For this review, use the dimensioned drawing (mm, ordinates from the lowest corner) and the shaded views. A direction names the side the tool comes from. Coordinates: 2 decimals unless noted, no trailing zeros. Loops run counter-clockwise (first coordinate to the right, second up) from the corner with the lowest first, then second, coordinate; pieces in that order, holes last. Notation, with made-up numbers: (6.5, 55.25) - (20.5, 55.25) arc R28 ccw to (20.5, 94.25) - close; hole circle Ø6 at (-13.5, -22.75). An arc over 180 degrees is marked (long way). Answer in a Markdown table with one row per item. Add a question column.
(1) We need section D-D on x = 12.5. Write out the cut boundary in (y, z), plus the area to 3 significant figures.
(2) For line 1 along X through (y, z) = (10, 34); line 2 along Z through (x, y) = (22.75, 9.75); line 3 along Z through (x, y) = (17.25, 8), list the stretches that pass through material, from the lowest coordinate up.
(3) We need section A-A on z = 32. Write out the cut boundary in (x, y).
(4) We need section C-C on y = 12.5. Write out the cut boundary in (x, z), plus the area to 3 significant figures.
(5) Machinability: for the marked faces 1, 2, 3, 4 and 5, which of the approach directions +Z, -Z, +X, -X, +Y, -Y give a long, thin tool a straight path to every point of the face, cutting with its end or side? Answer none if there is none.
(6) Mouldability with a two-part tool opening along Z and no side actions: class the marked faces 6, 7, 8 and 9 as +Z half, -Z half, draft (parallel to the pull), parting line (faces both ways), or undercut.
(7) For P1, Ø2, axis at x = 20.5, z = 6, coming from the +Y side; P2, Ø2, axis at y = 11, z = 21, coming from the +X side; P3, Ø5.5, axis at y = 14, z = 34.5, coming from the +X side, all flat-tipped, find the tip position at first contact; note any pin that passes through.
(8) We need section B-B on x = 4. Write out the cut boundary in (y, z), plus the area to 3 significant figures.
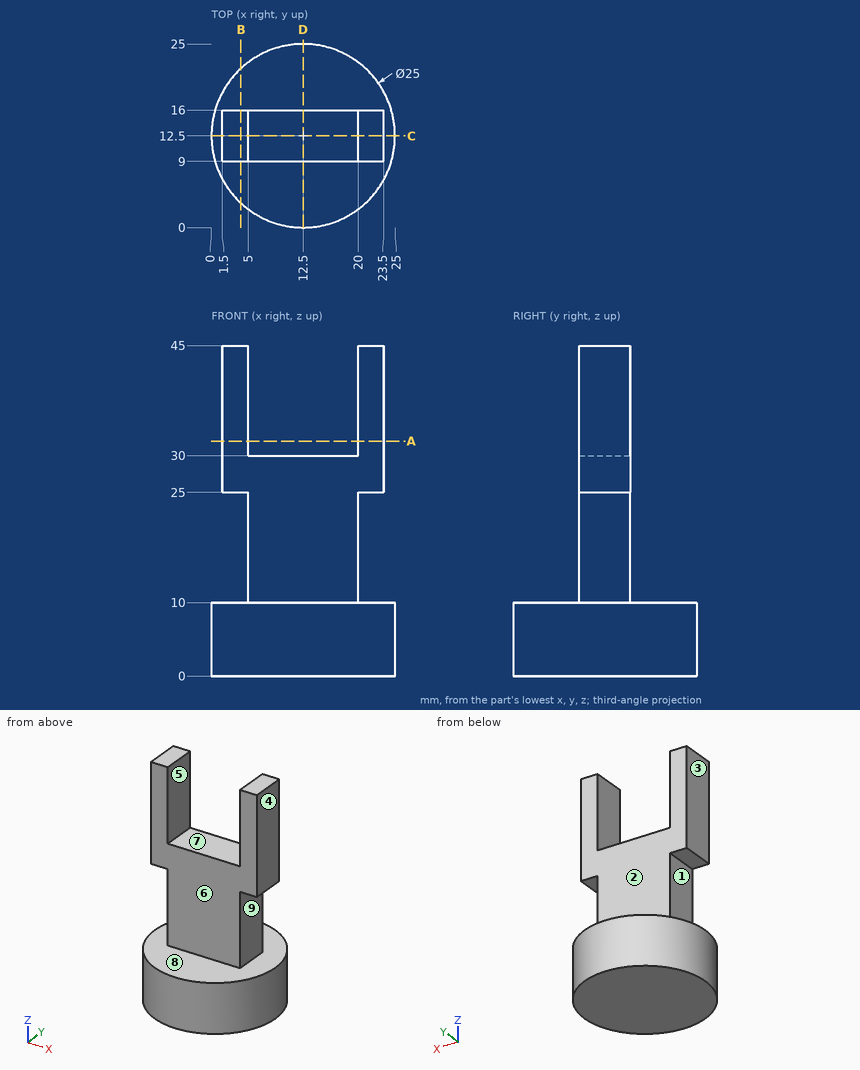
Outcome:
| question | item | result |
|---|---|---|
| 1 | outline | (0, 0) - (25, 0) - (25, 10) - (16, 10) - (16, 30) - (9, 30) - (9, 10) - (0, 10) - close |
| 1 | area | 390 mm² |
| 2 | line 1 | 1.5 to 5, 20 to 23.5 |
| 2 | line 2 | 0 to 10, 25 to 45 |
| 2 | line 3 | 0 to 10 |
| 3 | outline | (1.5, 9) - (5, 9) - (5, 16) - (1.5, 16) - close; (20, 9) - (23.5, 9) - (23.5, 16) - (20, 16) - close |
| 4 | outline | (0, 0) - (25, 0) - (25, 10) - (20, 10) - (20, 25) - (23.5, 25) - (23.5, 45) - (20, 45) - (20, 30) - (5, 30) - (5, 45) - (1.5, 45) - (1.5, 25) - (5, 25) - (5, 10) - (0, 10) - close |
| 4 | area | 690 mm² |
| 5 | face 1 | -X, +Y, -Y |
| 5 | face 2 | +Z, +X, -X, +Y |
| 5 | face 3 | +Z, -X, +Y, -Y |
| 5 | face 4 | +Z, +X, +Y, -Y |
| 5 | face 5 | +Z, +Y, -Y |
| 6 | face 6 | draft |
| 6 | face 7 | +Z half |
| 6 | face 8 | undercut |
| 6 | face 9 | undercut |
| 7 | P1 | y = 22.86 |
| 7 | P2 | x = 20 |
| 7 | P3 | x = 23.5 |
| 8 | outline | (3.33, 0) - (21.67, 0) - (21.67, 10) - (3.33, 10) - close; (9, 25) - (16, 25) - (16, 45) - (9, 45) - close |
| 8 | area | 323 mm² |
